Work out the finished part from the listing and answer in its coordinate system (mm). A direction names the side the tool comes from. Coordinates: 2 decimals unless noted, no trailing zeros. Write each loop counter-clockwise with the first axis right and the second up, starting at its lowest first coordinate (ties: lowest second). Pieces come first, ordered by that corner, then holes. Notation, with made-up numbers: (-38.5, 14.25) - (-22.5, 14.25) arc R11 ccw to (-22.5, 24.25) - close; hole circle Ø4 at (32, 26.25). An arc over 180 degrees is marked (long way). Use one line per item in the form item = value. Start each with the question number.
Item 1: A cutting plane is placed at D-D (y = 34). Write down the section's boundary in (x, z).
Item 2: A cutting plane is placed at A-A (x = -13). Write down the section's boundary in (y, z).
Item 3: Consider probe 1 along Y at (x, z) = (-5, 0.7); probe 2 along Y at (x, z) = (-16, 0.95); probe 3 along X at (y, z) = (19.5, 4). Determine where each line is inside the solid, lowest interval first.
Item 4: A cutting plane is placed at C-C (x = -16). Write down the section's boundary in (y, z), then the cut area to 3 significant figures.
Item 5: Given pin 1 (2.5 mm diameter, centred on x = -5, y = 5, fed in from -Z); pin 2 (6 mm diameter, centred on x = -14.5, y = 10.5, fed in from +Z); pin 3 (4.5 mm diameter, centred on y = 31.5, z = 7, fed in from -X); pin 4 (3 mm diameter, centred on y = 24, z = 1, fed in from -X), each flat-ended and moving along its own axis, determine where each tip first touches the part or whether it passes through.
Item 6: For faces 4 (the cylindrical face through (-0.86, 49.1, 1.32)), 5 (the cylindrical face through (-6.5, 25.1, 17.7)), 6 (the flat face through (-12, 10, 1)), determine the directions among +Z, -Z, +X, -X, +Y, -Y from which every point of the face is accessible in a straight line to the end or side of a thin tool.
Item 7: A cutting plane is placed at B-B (y = 45). Write down the section's boundary in (x, z).
Item 8: Determine the mould class of faces 1 (the flat face through (0, 25, 4)), 2 (the cylindrical face through (-1.479, 17.525, 6.766)), 3 (the cylindrical face through (-5, 43, 1)) for opening direction Y: released by +Y, released by -Y, zero draft, split by the parting line, or undercut.
from build123d import *

# Parameters (mm, degrees)
F0_R     = 2
F1_DEPTH = 2.6
F2_R     = 3.25
F3_DEPTH = 26
F4_R     = 3
F6_DEPTH = 3
F7_R     = 1


with BuildPart() as f1:
    # F0 (on Top) → F1 (new body)
    with BuildSketch(Plane.XY):
        Polygon((0, 50), (-20, 50), (-20, 40), (-6.5, 40), (-6.5, 10), (-20, 10), (-20, 0), (0, 0), align=None)
        with Locations((-16, 5)):
            Circle(F0_R, mode=Mode.SUBTRACT)
        with Locations((-5, 5)):
            Circle(F0_R, mode=Mode.SUBTRACT)
        with Locations((-16, 45)):
            Circle(F0_R, mode=Mode.SUBTRACT)
        with Locations((-5, 45)):
            Circle(F0_R, mode=Mode.SUBTRACT)
    extrude(amount=F1_DEPTH)

    # F2 (on face) → F3 (join)
    with BuildSketch(Plane.XY.offset(2.6)):
        with Locations((-3.25, 25)):
            Circle(F2_R)
    extrude(amount=F3_DEPTH)

    # F4
    f4_edges = [f1.edges().sort_by_distance(p)[0] for p in [
        (-20, 50, 1.3),
        (-20, 40, 1.3),
        (-20, 10, 1.3),
        (-20, 0, 1.3),
        (0, 50, 1.3),
        (0, 0, 1.3),
    ]]
    fillet(f4_edges, radius=F4_R)

    # F5 (on face) → F6 (join)
    with BuildSketch(Plane.YZ):
        with BuildLine():
            ThreePointArc((25, 17.891796), (19.263456, 8.336544), (9.708204, 2.6))
            Line((9.708204, 2.6), (25, 2.6))
            Line((25, 2.6), (40.291796, 2.6))
            ThreePointArc((40.291796, 2.6), (30.736544, 8.336544), (25, 17.891796))
        make_face()
    extrude(amount=-F6_DEPTH)

    # F7
    f7_edges = [f1.edges().sort_by_distance(p)[0] for p in [
        (-6.5, 25, 28.6),
    ]]
    fillet(f7_edges, radius=F7_R)


solid = f1.part
Answer:
q1.outline = (-6.5, 0) - (0, 0) - (0, 5.63) - (-3, 5.63) - (-3, 2.6) - (-6.5, 2.6) - close
q2.outline = (0, 0) - (10, 0) - (10, 2.6) - (0, 2.6) - close; (40, 0) - (50, 0) - (50, 2.6) - (40, 2.6) - close
q3.probe_1 = 0 to 3, 7 to 43, 47 to 50
q3.probe_2 = 0 to 3, 7 to 10, 40 to 43, 47 to 50
q3.probe_3 = -3 to 0
q4.outline = (0, 0) - (3, 0) - (3, 2.6) - (0, 2.6) - close; (7, 0) - (10, 0) - (10, 2.6) - (7, 2.6) - close; (40, 0) - (43, 0) - (43, 2.6) - (40, 2.6) - close; (47, 0) - (50, 0) - (50, 2.6) - (47, 2.6) - close
q4.area = 31.2 mm²
q5.pin_1 = through
q5.pin_2 = 2.6
q5.pin_3 = -3
q5.pin_4 = -6.5
q6.face_4 = +Z, -Z, +X, +Y
q6.face_5 = +Z
q6.face_6 = +Z, -Z, -X
q7.outline = (-20, 0) - (-18, 0) - (-18, 2.6) - (-20, 2.6) - close; (-14, 0) - (-7, 0) - (-7, 2.6) - (-14, 2.6) - close; (-3, 0) - (0, 0) - (0, 2.6) - (-3, 2.6) - close
q8.face_1 = zero draft
q8.face_2 = released by -Y
q8.face_3 = undercut
